Source: CAD feature listing. Evaluate the final solid. Frame: model axes, mm. Face numbers are marked on the shaded views. Coordinates: 2 decimals unless noted, no trailing zeros. Loops run counter-clockwise (first coordinate to the right, second up) from the corner with the lowest first, then second, coordinate; pieces in that order, holes last.
```python
from build123d import *

# Parameters (mm, degrees)
BASPROSKE_W         = 3
BASPROSKE_H         = 24
TOOTHCUT_DEPTH      = 35.073450075
TEETHCUTS_COUNT     = 10
TEETHCUTS_ANGLE     = 324
BORSKE_R            = 1.5
BORE_DEPTH          = 50.0000508
CUT_EXTRUDE1_DEPTH  = 10
BOSS_EXTRUDE1_DEPTH = 3
FILLET1_R           = 10
FILLET2_R           = 0.5


with BuildPart() as part:
    # BasProSke → Base-Revolve (revolve)
    with BuildSketch(Plane(origin=(0, 0, 0), x_dir=(1, 0, 0), z_dir=(0, 1, 0)), mode=Mode.PRIVATE) as base_revolve_sk:
        with Locations((1.5, 12)):
            Rectangle(BASPROSKE_W, BASPROSKE_H)
    revolve(base_revolve_sk.sketch.rotate(Axis((-10, 0, 0), (1, 0, 0)), 180), axis=Axis((-10, 0, 0), (1, 0, 0)))

    # TooCutSke → ToothCut (cut, through all)
    with BuildSketch(Plane(origin=(0, 0, 0), x_dir=(0, 0, -1), z_dir=(1, 0, 0))):
        with BuildLine():
            ThreePointArc((2.33803632, 14.815653451), (0, 14.999), (-2.33803632, 14.815653451))
            ThreePointArc((-2.33803632, 14.815653451), (-3.315013319, 19.654913653), (-6.946609122, 22.999227528))
            ThreePointArc((-6.946609122, 22.999227528), (0, 24.0254), (6.946609122, 22.999227528))
            ThreePointArc((6.946609122, 22.999227528), (3.315013319, 19.654913653), (2.33803632, 14.815653451))
        make_face()
    toothcut = extrude(amount=TOOTHCUT_DEPTH, mode=Mode.SUBTRACT)

    # TeethCuts: ToothCut ×10 about axis
    teethcuts_axis = Axis((-10, 0, 0), (1, 0, 0))
    for i in range(1, TEETHCUTS_COUNT):
        add(toothcut.rotate(teethcuts_axis, i * TEETHCUTS_ANGLE / (TEETHCUTS_COUNT - 1)), mode=Mode.SUBTRACT)

    # BorSke → Bore (cut, symmetric)
    with BuildSketch(Plane(origin=(0, 0, 0), x_dir=(0, 0, -1), z_dir=(1, 0, 0))):
        with Locations(Location((0, 0, 0), (0, 0, 180))):
            Circle(BORSKE_R)
    extrude(amount=BORE_DEPTH, both=True, mode=Mode.SUBTRACT)

    # Sketch1 → Cut-Extrude1 (cut)
    with BuildSketch(Plane.ZY):
        Polygon((6.816911485, -13.360378693), (2.33803632, -14.815653451), (0, -15.575327501), (3.846423881, -27.413402957), (12.603452521, -24.568071871), (8.75702864, -12.729996416), align=None)
    extrude(amount=-CUT_EXTRUDE1_DEPTH, mode=Mode.SUBTRACT)

    # Sketch2 → Boss-Extrude1 (add)
    with BuildSketch(Plane.ZY):
        Polygon((11.666327165, -43.525180612), (16.145202329, -42.069905854), (6.816911485, -13.360378693), (2.33803632, -14.815653451), align=None)
        Polygon((13.905764747, -53.929068958), (9.648574383, -53.929068958), (11.666327165, -43.525180612), (16.145202329, -42.069905854), align=None)
    extrude(amount=-BOSS_EXTRUDE1_DEPTH)

    # Fillet1
    fillet1_edges = [part.edges().sort_by_distance(p)[0] for p in [
        (1.5, -43.525180612, 11.666327165),
        (1.5, -42.069905854, 16.145202329),
    ]]
    fillet(fillet1_edges, radius=FILLET1_R)

    # Fillet2
    fillet2_edges = [part.edges().sort_by_distance(p)[0] for p in [
        (1.5, -53.929068958, 13.905764747),
        (1.5, -53.929068958, 9.648574383),
    ]]
    fillet(fillet2_edges, radius=FILLET2_R)


solid = part.part
```
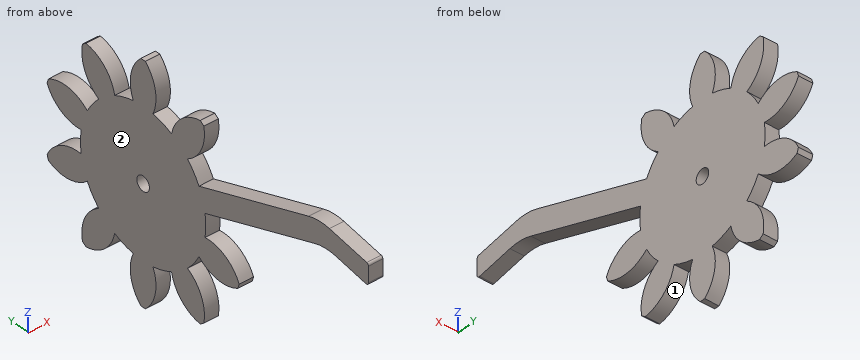
Q1. Section query A-A on z = 0. Return the cut outline in (x, y).
Q2. Material intervals for line 1 along Y through (x, z) = (1.05, 0); line 2 along Y through (x, z) = (0.9, -15.5); line 3 along Y through (x, z) = (0.85, -19), sorted ascending.
Q3. Draft query along Y for the marked faces 1 and 2. Return one class per face: released by +Y, released by -Y, zero draft, split by the parting line, or undercut.
Q4. First-contact query: pin 1 Ø1.5 at (x, z) = (1.5, -3.5) entering from +Y; pin 2 Ø1 at (x, y) = (2, -35) entering from +Z. Flat tips, straight axial feed; report the tip coordinate or a pass-through.
Q5. Section query B-B on z = 20.5. Return the cut outline in (x, y), then the cut area to 3 significant figures.
Resolved:
1. outline: (0, -15) - (3, -15) - (3, -1.5) - (0, -1.5) - close; (0, 1.5) - (3, 1.5) - (3, 15) - (0, 15) - close
2. line 1: y = -15 to -1.5, 1.5 to 15
2. line 2: y = -14.41 to -7.56, -2.63 to 2.63, 7.56 to 14.41
2. line 3: y = -14.55 to -11.2, -3.03 to 3.03, 11.2 to 14.55
3. face 1: undercut
3. face 2: zero draft
4. pin 1: stops at y = 20.98
4. pin 2: stops at z = 14.01
5. outline: (0, -2.72) - (3, -2.72) - (3, 2.72) - (0, 2.72) - close
5. area: 16.3 mm2
